```python
from build123d import *

# Parameters (mm, degrees)
EXTRUDE_THIN3_DEPTH    = 21.59
CONVERT_SOLID1_START   = -21.59
CONVERT_SOLID1_DEPTH   = 43.18
CONVERT_SOLID1_2_DEPTH = 43.18


# Read off the part's stored shape, not the designer's step: Convert-Solid1
with BuildPart() as part:
    # Sketch6 → Extrude-Thin3 (new, symmetric)
    with BuildSketch(Plane.XY):
        Polygon((15.113, 2.159), (17.653, 2.159), (17.653, 0), (-17.653, 0), (-17.653, 2.159), (-15.113, 2.159), (-15.113, 2.559), (-18.053, 2.559), (-18.053, -0.4), (18.053, -0.4), (18.053, 2.559), (15.113, 2.559), align=None)
    extrude(amount=EXTRUDE_THIN3_DEPTH, both=True)

    # Convert-Solid1 outline → Convert-Solid1 (cut)
    with BuildSketch(Plane.XY.offset(CONVERT_SOLID1_START)):
        with BuildLine():
            Line((-18.053, 2.559), (-18.053, 1.959))
            ThreePointArc((-18.053, 1.959), (-17.877264, 2.383264), (-17.453, 2.559))
            Line((-17.453, 2.559), (-18.053, 2.559))
        make_face()
        with BuildLine():
            Line((-18.053, -0.4), (-17.453, -0.4))
            ThreePointArc((-17.453, -0.4), (-17.877264, -0.224264), (-18.053, 0.2))
            Line((-18.053, 0.2), (-18.053, -0.4))
        make_face()
        with BuildLine():
            Line((18.053, -0.4), (18.053, 0.2))
            ThreePointArc((18.053, 0.2), (17.877264, -0.224264), (17.453, -0.4))
            Line((17.453, -0.4), (18.053, -0.4))
        make_face()
        with BuildLine():
            ThreePointArc((17.453, 2.559), (17.877264, 2.383264), (18.053, 1.959))
            Line((18.053, 1.959), (18.053, 2.559))
            Line((18.053, 2.559), (17.453, 2.559))
        make_face()
    extrude(amount=CONVERT_SOLID1_DEPTH, mode=Mode.SUBTRACT)

    # Convert-Solid1 2 outline → Convert-Solid1 2 (add)
    with BuildSketch(Plane.XY.offset(CONVERT_SOLID1_START)):
        with BuildLine():
            Line((-17.653, 2.159), (-17.653, 1.959))
            ThreePointArc((-17.653, 1.959), (-17.594421, 2.100421), (-17.453, 2.159))
            Line((-17.453, 2.159), (-17.653, 2.159))
        make_face()
        with BuildLine():
            Line((-17.653, 0), (-17.453, 0))
            ThreePointArc((-17.453, 0), (-17.594421, 0.058579), (-17.653, 0.2))
            Line((-17.653, 0.2), (-17.653, 0))
        make_face()
        with BuildLine():
            Line((17.653, 0), (17.653, 0.2))
            ThreePointArc((17.653, 0.2), (17.594421, 0.058579), (17.453, 0))
            Line((17.453, 0), (17.653, 0))
        make_face()
        with BuildLine():
            ThreePointArc((17.453, 2.159), (17.594421, 2.100421), (17.653, 1.959))
            Line((17.653, 1.959), (17.653, 2.159))
            Line((17.653, 2.159), (17.453, 2.159))
        make_face()
    extrude(amount=CONVERT_SOLID1_2_DEPTH)


solid = part.part
```
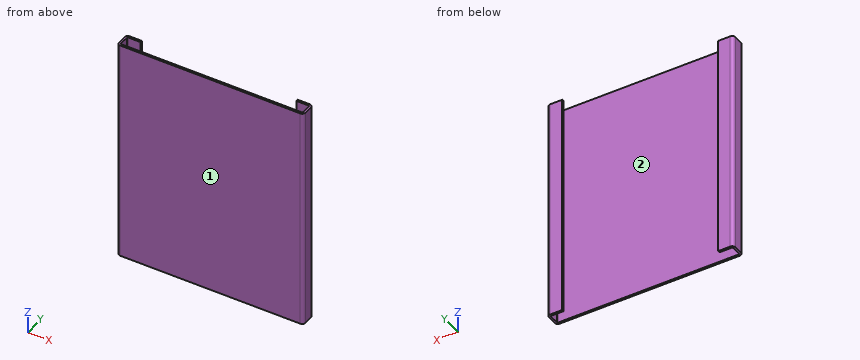
Check sheet for the modelled part. Datum: model origin and axes. Units: mm. Face numbers are marked on the shaded views. Coordinates: 2 decimals unless noted, no trailing zeros. Loops run counter-clockwise (first coordinate to the right, second up) from the corner with the lowest first, then second, coordinate; pieces in that order, holes last.
1) Material ranges on probe 1 along X at (y, z) = (1.1, -7.5); probe 2 along Y at (x, z) = (16.5, 14), recorded low to high.
2) Sectioned sample at B-B (z = -17.5). Record the boundary of the cut face in (x, y).
3) Gauge pin test, flat ends, axial feed: pin 1 (6 mm diameter, centred on x = -14, z = -4.5, fed in from +Y); pin 2 (10 mm diameter, centred on x = 8, z = 5, fed in from +Y). Record the tip position at first contact, or that the pin passes through.
4) Sectioned sample at C-C (x = 2.5). Record the boundary of the cut face in (y, z), and give its area (3 significant figures).
5) Release check for a two-part mould opening along X. For the marked faces 1 and 2 record: released by +X, released by -X, zero draft, split by the parting line, or undercut.
6) Sectioned sample at A-A (y = 1.35). Record the boundary of the cut face in (x, z).
Check sheet entries:
1. probe 1: x = -18.05 to -17.65, 17.65 to 18.05
1. probe 2: y = -0.4 to 0, 2.16 to 2.56
2. outline: (-18.05, 0.2) arc R0.6 ccw to (-17.45, -0.4) - (17.45, -0.4) arc R0.6 ccw to (18.05, 0.2) - (18.05, 1.96) arc R0.6 ccw to (17.45, 2.56) - (15.11, 2.56) - (15.11, 2.16) - (17.45, 2.16) arc R0.2 cw to (17.65, 1.96) - (17.65, 0.2) arc R0.2 cw to (17.45, 0) - (-17.45, 0) arc R0.2 cw to (-17.65, 0.2) - (-17.65, 1.96) arc R0.2 cw to (-17.45, 2.16) - (-15.11, 2.16) - (-15.11, 2.56) - (-17.45, 2.56) arc R0.6 ccw to (-18.05, 1.96) - close
3. pin 1: stops at y = 2.56
3. pin 2: stops at y = 0
4. outline: (-0.4, -21.59) - (0, -21.59) - (0, 21.59) - (-0.4, 21.59) - close
4. area: 17.3 mm2
5. face 1: zero draft
5. face 2: undercut
6. outline: (-18.05, -21.59) - (-17.65, -21.59) - (-17.65, 21.59) - (-18.05, 21.59) - close; (17.65, -21.59) - (18.05, -21.59) - (18.05, 21.59) - (17.65, 21.59) - close
